```python
from build123d import *

# Parameters (mm, degrees)
F0_W     = 30
F0_H     = 115
F0_H_2   = 150
F0_W_2   = 5
F0_W_3   = 160
F1_DEPTH = 3


with BuildPart() as f1:
    # F0 (on Front) → F1 (new body)
    with BuildSketch(Plane.XZ):
        with Locations((-95, 132.5)):
            Rectangle(F0_W, F0_H)
        with Locations((-95, 0)):
            Rectangle(F0_W, F0_H_2)
        with Locations((-112.5, 132.5)):
            Rectangle(F0_W_2, F0_H)
        Rectangle(F0_W_3, F0_H_2)
        with BuildLine():
            Line((-80, 190), (-80, 75))
            add(Edge.make_bspline(
                [(-41.8714651341, 178.0006884036), (-80, 180.026688963), (-80, 110.9410823158), (-80, 75)],
                knots=[0, 0, 0, 0, 109.8313570099, 109.8313570099, 109.8313570099, 109.8313570099], degree=3))
            Line((-41.8714651341, 178.0006884036), (-42, 190))
            Line((-42, 190), (-60, 190))
            Line((-60, 190), (-80, 190))
        make_face()
        Polygon((-110, 215), (-110, 190), (-80, 190), (-60, 190), (-60, 215), align=None)
        with Locations((95, 132.5)):
            Rectangle(F0_W, F0_H)
        with Locations((95, 0)):
            Rectangle(F0_W, F0_H_2)
        with BuildLine():
            add(Edge.make_bspline(
                [(41.8714651341, 178.0006884036), (80, 180.026688963), (80, 110.9410823158), (80, 75)],
                knots=[0, 0, 0, 0, 109.8313570099, 109.8313570099, 109.8313570099, 109.8313570099], degree=3))
            Line((80, 75), (80, 190))
            Line((80, 190), (60, 190))
            Line((60, 190), (42, 190))
            ThreePointArc((42, 190), (35.9360767688, 184.0646116347), (41.8714651341, 178.0006884036))
        make_face()
        with BuildLine():
            Line((-42, 190), (-41.8714651341, 178.0006884036))
            ThreePointArc((-41.8714651341, 178.0006884036), (-35.9360767688, 184.0646116347), (-42, 190))
        make_face()
        with Locations((112.5, 132.5)):
            Rectangle(F0_W_2, F0_H)
        Polygon((60, 190), (80, 190), (110, 190), (110, 215), (60, 215), align=None)
    extrude(amount=F1_DEPTH)


solid = f1.part
```
Here's how the part is built. I have some questions about the finished solid (model axes, mm). A direction names the side the tool comes from. Round coordinates to 2 decimals unless told otherwise and drop trailing zeros. Write each loop counter-clockwise with the first axis right and the second up, starting at its lowest first coordinate (ties: lowest second). Pieces come first, ordered by that corner, then holes. Notation, with made-up numbers: M 43.25,15.5 L 55.25,15.5 A12 cw 55.25,34.5 Z; hole C 43,-10.5 d4. An arc over 180 degrees is marked long. Answer as CSV lines item,"result". Start each with the question number.
1. Thinking about a two-plate mould opening in X: for faces 1 (the flat face through (-2, 0, 40)), 2 (the cylindrical face through (35.94, -1.48, 184.2)), which applies, released by +X, released by -X, zero draft, split by the parting line, or undercut?
2. On a 3-axis mill with a long thin cutter (end or side, diameter ignored), from which of +Z, -Z, +X, -X, +Y, -Y can I reach the whole of each face in a straight line? I mean faces 3 (the cylindrical face through (-35.936, -1.479, 183.933)), 4 (the flat face through (-2, -3, 40)). Say none if no direction works.
3. Suppose I cut it at A-A on z = 46. Write out the boundary of the cut face in (x, y), then the cut area to 3 significant figures.
4. I need wall thicknesses on probe 1 along X at (y, z) = (-1.9, 142); probe 2 along Z at (x, y) = (-46, -1.55); probe 3 along X at (y, z) = (-1.75, 85). Which ranges of each line are inside material? Lowest first, please.
5. I'm going to push flat-ended pins straight in: pin 1 Ø1.5 at (y, z) = (-1, -26) entering from +X; pin 2 Ø1.5 at (x, y) = (112, -1) entering from +Z; pin 3 Ø1.5 at (x, y) = (113, -2) entering from -Z. Where does each tip first touch, or does it pass through?
6. Suppose I cut it at B-B on x = 31. Write out the boundary of the cut face in (y, z).
Check result:
1,face 1,"zero draft"
1,face 2,"undercut"
2,face 3,"+Y, -Y"
2,face 4,"+Z, -Z, +X, -X, -Y"
3,outline,"M -110,-3 L 110,-3 L 110,0 L -110,0 Z"
3,area,"660 mm2"
4,probe 1,"x = -115 to -74.95, 74.95 to 115"
4,probe 2,"z = -75 to 75, 177.93 to 190"
4,probe 3,"x = -115 to -79.98, 79.98 to 115"
5,pin 1,"stops at x = 110"
5,pin 2,"stops at z = 190"
5,pin 3,"stops at z = 75"
6,outline,"M -3,-75 L 0,-75 L 0,75 L -3,75 Z"
